Input: part model. Units: mm. Frame: model coordinates. A direction names the side the tool comes from. Coordinates: 2 decimals unless noted, no trailing zeros. Order: outer loops, then holes, each group sorted by start corner. A loop starts at its lowest first (then second) coordinate and runs counter-clockwise, first axis right, second up. Notation, with made-up numbers: M 15.25,55 L 22.25,55 A21 ccw 22.25,93 Z; hole C 77,52.5 d8. An arc over 180 degrees is marked long. One line per item, written item: value.
```python
from build123d import *

# Parameters (mm, degrees)
SKETCH2_R                = 28.575
SKETCH2_R_2              = 11.1125
BOSS_EXTRUDE1_DEPTH      = 6.35
BOSS_EXTRUDE2_DEPTH      = 3.175
BOSS_EXTRUDE2_DEPTH_BACK = 1.524
SKETCH3_W                = 9.954249144
SKETCH3_H                = 25.4
BOSS_EXTRUDE3_DEPTH      = 11.176
SKETCH4_W                = 1.247460898
SKETCH4_H                = 31.75
CUT_EXTRUDE1_DEPTH       = 197.090385348
FILLET2_R                = 3.175
FILLET4_R                = 3.175
FILLET7_R                = 1.5875
SKETCH5_R                = 28.575
CUT_EXTRUDE2_DEPTH       = 197.296936937
SKETCH6_R                = 28.575
BOSS_EXTRUDE4_DEPTH      = 4.699
F_3_8_CLEARANCE_HOLE1_D  = 10.31748
FILLET9_R                = 50.8
F_4_CLEARANCE_HOLE1_D    = 3.4544
CUT_EXTRUDE3_DEPTH       = 1.6002


with BuildPart() as part:
    # Sketch2 → Boss-Extrude1 (new body)
    with BuildSketch(Plane(origin=(0, 0, 0), x_dir=(0, 0, -1), z_dir=(1, 0, 0))):
        Circle(SKETCH2_R)
        Circle(SKETCH2_R_2, mode=Mode.SUBTRACT)
    extrude(amount=-BOSS_EXTRUDE1_DEPTH)

    # Sketch2<5> → Boss-Extrude2 (add, two sides: drawn at the far end of the back side and taken through both)
    with BuildSketch(Plane(origin=(0, 0, 0), x_dir=(0, 0, -1), z_dir=(1, 0, 0)).offset(-BOSS_EXTRUDE2_DEPTH_BACK)):
        with BuildLine():
            Line((11.55989339, 26.132345662), (4.977124572, 193.675))
            Line((4.977124572, 193.675), (0, 193.675))
            Line((0, 193.675), (0, 28.575))
            ThreePointArc((0, 28.575), (5.907573431, 27.957668021), (11.55989339, 26.132345662))
        make_face()
        with BuildLine():
            Line((0, 28.575), (0, 193.675))
            Line((0, 193.675), (-4.977124572, 193.675))
            Line((-4.977124572, 193.675), (-11.55989339, 26.132345662))
            ThreePointArc((-11.55989339, 26.132345662), (-5.907573431, 27.957668021), (0, 28.575))
        make_face()
    extrude(amount=BOSS_EXTRUDE2_DEPTH + BOSS_EXTRUDE2_DEPTH_BACK)

    # Sketch3 → Boss-Extrude3 (add)
    with BuildSketch(Plane(origin=(3.175, 0, 0), x_dir=(0, 0, -1), z_dir=(1, 0, 0))):
        with Locations((0, 180.975)):
            Rectangle(SKETCH3_W, SKETCH3_H)
    extrude(amount=BOSS_EXTRUDE3_DEPTH)

    # Sketch4 → Cut-Extrude1 (cut, through all)
    with BuildSketch(Plane(origin=(3.175, 0, 0), x_dir=(0, 0, -1), z_dir=(1, 0, 0))):
        with Locations((-5.600855021, 177.8)):
            Rectangle(SKETCH4_W, SKETCH4_H)
        with Locations((5.600855021, 177.8)):
            Rectangle(SKETCH4_W, SKETCH4_H)
    extrude(amount=-CUT_EXTRUDE1_DEPTH, mode=Mode.SUBTRACT)

    # Fillet2
    # the kernel refuses this fillet: 3.175 mm, written as the material it takes off along each edge
    with BuildSketch(Plane(origin=(9.358070531, 161.925, 6.22458547), x_dir=(0, -0.999229036240723, 0.039259815759068305), z_dir=(-1, 0, 0))) as fillet2_piece_1:
        with BuildLine():
            CenterArc((2.473228212, -3.175), FILLET2_R, 90, 52.598124578)
            Line((-0.048975085, -1.24649915), (-0.099419151, -1.207929133))
            ThreePointArc((-0.099419151, -1.207929133), (-0.087938586, -0.620756577), (-0.063451044, 0.002492998))
            Line((-0.063451044, 0.002492998), (0, 0.0635))
            Line((0, 0.0635), (2.473228212, 0.0635))
            Line((2.473228212, 0.0635), (2.473228212, 0))
        make_face()
    extrude(amount=17.065141061, mode=Mode.SUBTRACT)
    with BuildSketch(Plane(origin=(9.358070531, 161.925, -6.22458547), x_dir=(0, 0, 1), z_dir=(-1, 0, 0))) as fillet2_piece_2:
        with BuildLine():
            CenterArc((3.075453706, -2.595971358), FILLET2_R, 125.151875422, 52.598124578)
            Line((-0.097098484, -2.471321443), (-0.160549528, -2.468828445))
            Line((-0.160549528, -2.468828445), (-0.063451044, 0.002492998))
            Line((-0.063451044, 0.002492998), (0, 0.0635))
            ThreePointArc((0, 0.0635), (0.623730449, 0.0635), (1.210901041, 0.051919427))
            Line((1.210901041, 0.051919427), (1.247460897, 0))
        make_face()
    extrude(amount=17.065141061, mode=Mode.SUBTRACT)

    # Fillet4
    fillet4_edges = [part.edges().sort_by_distance(p)[0] for p in [
        (0.8255, 161.925, 4.977124572),
        (0.8255, 161.925, -4.977124572),
    ]]
    fillet(fillet4_edges, radius=FILLET4_R)

    # Fillet7
    fillet7_edges = [part.edges().sort_by_distance(p)[0] for p in [
        (6.4135, 193.675, 4.977124572),
        (6.4135, 193.675, -4.977124572),
        (-1.524, 193.675, 0),
        (8.763, 168.275, 4.977124572),
        (8.763, 168.275, -4.977124572),
        (14.351, 193.675, 0),
        (14.351, 180.975, 4.977124572),
        (14.351, 168.275, 0),
        (14.351, 180.975, -4.977124572),
    ]]
    fillet(fillet7_edges, radius=FILLET7_R)

    # Sketch5 → Cut-Extrude2 (cut, through all)
    with BuildSketch(Plane(origin=(0, 0, 0), x_dir=(0, 0, -1), z_dir=(1, 0, 0))):
        Circle(SKETCH5_R)
    extrude(amount=-CUT_EXTRUDE2_DEPTH, mode=Mode.SUBTRACT)

    # Sketch6 → Boss-Extrude4 (add)
    with BuildSketch(Plane(origin=(3.175, 0, 0), x_dir=(0, 0, -1), z_dir=(1, 0, 0))):
        Circle(SKETCH6_R)
    extrude(amount=-BOSS_EXTRUDE4_DEPTH)

    # 3/8 Clearance Hole1 (through all)
    with Locations(Plane(origin=(3.175, 0, 0), x_dir=(0, 0, -1), z_dir=(1, 0, 0))):
        with Locations((0, 0)):
            Hole(F_3_8_CLEARANCE_HOLE1_D / 2)

    # Fillet9
    fillet9_edges = [part.edges().sort_by_distance(p)[0] for p in [
        (0.8255, 26.132345662, -11.55989339),
        (0.8255, 26.132345662, 11.55989339),
    ]]
    fillet(fillet9_edges, radius=FILLET9_R)

    # #4 Clearance Hole1 (through all)
    with Locations(Plane(origin=(3.175, 0, 0), x_dir=(0, 0, -1), z_dir=(1, 0, 0))):
        with Locations((0, 49.88728048)):
            Hole(F_4_CLEARANCE_HOLE1_D / 2)

    # Sketch11 → Cut-Extrude3 (cut)
    with BuildSketch(Plane(origin=(3.175, 0, 0), x_dir=(0, 0, -1), z_dir=(1, 0, 0))):
        Polygon((-1.382344076, 47.492990308), (1.382344076, 47.492990308), (2.764688151, 49.88728048), (1.382344076, 52.281570653), (-1.382344076, 52.281570653), (-2.764688151, 49.88728048), align=None)
    extrude(amount=-CUT_EXTRUDE3_DEPTH, mode=Mode.SUBTRACT)


solid = part.part
```
(1) Cut plane A-A on y = 0. Output: boundary loops of the cut face in (x, z) (3 decimals).
Data:
outline: M -1.524,-28.575 L 3.175,-28.575 L 3.175,-5.159 L -1.524,-5.159 Z; M -1.524,5.159 L 3.175,5.159 L 3.175,28.575 L -1.524,28.575 Z
(2) Cut plane C-C on y = 136. Output: boundary loops of the cut face in (x, z) (3 decimals).
Data:
outline: M -1.524,-7.243 L 3.175,-7.243 L 3.175,7.243 L -1.524,7.243 Z
(3) Cut plane B-B on x = 10.5. Output: boundary loops of the cut face in (y, z) (1 decimal), plus the area to 3 significant figures.
Data:
outline: M 168.3,-3.4 A1.6 ccw 169.9,-5 L 192.1,-5 A1.6 ccw 193.7,-3.4 L 193.7,3.4 A1.6 ccw 192.1,5 L 169.9,5 A1.6 ccw 168.3,3.4 Z
area: 251 mm2
(4) First-contact query: pin 1 (5 mm diameter, centred on x = 2.5, y = 48.5, fed in from -Z); pin 2 (3 mm diameter, centred on x = 0.5, z = 22, fed in from +Y); pin 3 (1.4 mm diameter, centred on y = 49.5, z = -1.5, fed in from +X). Flat tips, straight axial feed; report the tip coordinate or a pass-through.
Data:
pin 1: stops at z = -10.83
pin 2: stops at y = 20.18
pin 3: stops at x = 1.57
(5) Cut plane D-D on z = 15.5. Output: boundary loops of the cut face in (x, y) (3 decimals).
Data:
outline: M -1.524,-24.006 L 3.175,-24.006 L 3.175,28.582 L -1.524,28.582 Z
(6) Draft query along Y for faces 5 (the flat face through (3.175, 50, -6)), 6 (the flat face through (6, 193.675, 0)), 7 (the flat face through (1.575, 52, -1)). Return one class per face: released by +Y, released by -Y, zero draft, split by the parting line, or undercut.
Data:
face 5: zero draft
face 6: released by +Y
face 7: undercut
(7) Access query for faces 1 (the flat face through (6, 181, -4.977)), 2 (the flat face through (8, 168.275, 0)), 3 (the flat face through (6, 181, 4.977)), 4 (the flat face through (14.351, 181, 0)). Directions: +Z, -Z, +X, -X, +Y, -Y. A direction counts if a zero-diameter tool reaches every point of the face in a straight line with its end or side. Return the directions, or none.
Data:
face 1: -Z, +X, -X, +Y
face 2: +Z, -Z, +X, -Y
face 3: +Z, +X, -X, +Y
face 4: +Z, -Z, +X, +Y, -Y
(8) Ray query, line 1 (Y direction, x = -0.3, z = 0) (3 decimals); line 2 (Y direction, x = 2.25, z = 0) (3 decimals); line 3 (X direction, y = 11.5, z = 15) (3 decimals). Return the intervals inside material, ascending. Write a range as from..to.
Data:
line 1: y = -28.575..-5.159, 5.159..48.16, 51.614..193.633
line 2: y = -28.575..-5.159, 5.159..47.493, 52.282..193.675
line 3: x = -1.524..3.175
